from build123d import *

# Parameters (mm, degrees)
F0_W     = 103
F0_H     = 103
F1_DEPTH = 3
F2_W     = 0.95
F2_H     = 19
F2_W_2   = 19
F2_H_2   = 0.95
F3_DEPTH = 5


with BuildPart() as f1:
    # F0 (on Top) → F1 (new body)
    with BuildSketch(Plane.XY):
        with Locations((51.5, 51.5)):
            Rectangle(F0_W, F0_H)
    extrude(amount=F1_DEPTH)

    # F2 (on face) → F3 (join)
    with BuildSketch(Plane.XY.offset(3)):
        with Locations((1.525, 11.5)):
            Rectangle(F2_W, F2_H)
        Polygon((2, 2), (1.05, 2), (1.05, 1.05), (21.05, 1.05), (21.05, 2), align=None)
        Polygon((101, 2), (81.95, 2), (81.95, 1.05), (101.95, 1.05), (101.95, 2), align=None)
        with Locations((101.475, 11.5)):
            Rectangle(F2_W, F2_H)
        Polygon((101.95, 81.95), (101.95, 101.95), (101, 101.95), (101, 101), (101, 81.95), align=None)
        with Locations((91.5, 101.475)):
            Rectangle(F2_W_2, F2_H_2)
        Polygon((21.05, 101.95), (1.05, 101.95), (1.05, 101), (2, 101), (21.05, 101), align=None)
        with Locations((1.525, 91.5)):
            Rectangle(F2_W, F2_H)
    extrude(amount=F3_DEPTH)


solid = f1.part
Design review of the part built by this model. Coordinates are the model's own, in mm. A direction names the side the tool comes from. Coordinates: 2 decimals unless noted, no trailing zeros. Write each loop counter-clockwise with the first axis right and the second up, starting at its lowest first coordinate (ties: lowest second). Pieces come first, ordered by that corner, then holes. Notation, with made-up numbers: (43.25, 67.25) - (96.25, 67.25) arc R25 cw to (96.25, 92.25) - close; hole circle Ø5 at (49.5, 4). An arc over 180 degrees is marked (long way). One line per item, written item: value.
1) For faces 4 (the face through (101.95, 92, 5)), 5 (the face through (92, 101.95, 5)), 6 (the face through (6.6, 1.5, 8)), 7 (the face through (92, 1.05, 5)), 8 (the face through (2, 11, 5)), list the 3-axis set-ups (+Z, -Z, +X, -X, +Y, -Y) from which the entire face can be reached by the end or side of a thin tool; tool diameter is ignored.
Answer sheet:
face 4: +Z, +X, +Y, -Y
face 5: +Z, +X, -X, +Y
face 6: +Z, +X, -X, +Y, -Y
face 7: +Z, +X, -X, -Y
face 8: +Z
2) To check wall thickness, follow probe 1 along Y at (x, z) = (85.5, 6.75); probe 2 along Z at (x, y) = (60.5, 51.5). State the ranges of each line that lie inside material, in increasing order.
Answer sheet:
probe 1: y = 1.05 to 2, 101 to 101.95
probe 2: z = 0 to 3
3) Add section C-C (x = 22.5). State the section outline as (y, z) points, plus the area to 3 significant figures.
Answer sheet:
outline: (0, 0) - (103, 0) - (103, 3) - (0, 3) - close
area: 309 mm2
4) Add section B-B (y = 89.5). State the section outline as (x, z) points.
Answer sheet:
outline: (0, 0) - (103, 0) - (103, 3) - (101.95, 3) - (101.95, 8) - (101, 8) - (101, 3) - (2, 3) - (2, 8) - (1.05, 8) - (1.05, 3) - (0, 3) - close
5) Insertion check: pin 1 (2.5 mm diameter, centred on y = 87, z = 6.5, fed in from -X); pin 2 (1 mm diameter, centred on x = 27.5, y = 64, fed in from +Z); pin 3 (4 mm diameter, centred on y = 90, z = 6.5, fed in from +X). Each pin has a flat end and moves straight along its axis. Give the tip position at first contact, or say it passes through.
Answer sheet:
pin 1: stops at x = 1.05
pin 2: stops at z = 3
pin 3: stops at x = 101.95
6) Mouldability with a two-part tool opening along Y and no side actions: class faces 1 (the face through (11, 101.95, 5)), 2 (the face through (101, 92, 5)), 3 (the face through (6.6, 101.6, 8)) as +Y half, -Y half, draft (parallel to the pull), parting line (faces both ways), or undercut.
Answer sheet:
face 1: +Y half
face 2: undercut
face 3: draft
7) Add section A-A (z = 4.5). State the section outline as (x, y) points, plus the area to 3 significant figures.
Answer sheet:
outline: (1.05, 1.05) - (21.05, 1.05) - (21.05, 2) - (2, 2) - (2, 21) - (1.05, 21) - close; (1.05, 82) - (2, 82) - (2, 101) - (21.05, 101) - (21.05, 101.95) - (1.05, 101.95) - close; (81.95, 1.05) - (101.95, 1.05) - (101.95, 21) - (101, 21) - (101, 2) - (81.95, 2) - close; (82, 101) - (101, 101) - (101, 81.95) - (101.95, 81.95) - (101.95, 101.95) - (82, 101.95) - close
area: 148 mm2
